For this review, take the finished solid that the model builds, in its own axes (mm). Round coordinates to 2 decimals unless told otherwise and drop trailing zeros. Order: outer loops, then holes, each group sorted by start corner. A loop starts at its lowest first (then second) coordinate and runs counter-clockwise, first axis right, second up. Notation, with made-up numbers: M 61.5,73.25 L 101.5,73.25 A14 cw 101.5,95.25 Z; hole C 31,28 d6. An arc over 180 degrees is marked long. Answer as a JSON object with one key per item and string values.
from build123d import *

# Parameters (mm, degrees)
ESQUISSE1_W        = 100
ESQUISSE1_H        = 82
ESQUISSE1_R        = 1.35
BOSS_EXTRU_1_DEPTH = 2


with BuildPart() as part:
    # Esquisse1 → Boss.-Extru.1 (new body)
    with BuildSketch(Plane.XY.offset(50.5)):
        with Locations((9.361165235, -54.8)):
            Rectangle(ESQUISSE1_W, ESQUISSE1_H)
        with Locations((-36.138834765, -91.3)):
            Circle(ESQUISSE1_R, mode=Mode.SUBTRACT)
        with Locations((-36.138834765, -18.3)):
            Circle(ESQUISSE1_R, mode=Mode.SUBTRACT)
        with Locations((38.861165235, -91.3)):
            Circle(ESQUISSE1_R, mode=Mode.SUBTRACT)
        with Locations((38.861165235, -18.3)):
            Circle(ESQUISSE1_R, mode=Mode.SUBTRACT)
    extrude(amount=BOSS_EXTRU_1_DEPTH)


solid = part.part
1) Add section A-A on y = -91.3. State the section outline as (x, z) points.
Geometry check:
{"outline": "M -40.64,50.5 L -37.49,50.5 L -37.49,52.5 L -40.64,52.5 Z; M -34.79,50.5 L 37.51,50.5 L 37.51,52.5 L -34.79,52.5 Z; M 40.21,50.5 L 59.36,50.5 L 59.36,52.5 L 40.21,52.5 Z"}
2) Insertion check: P1, Ø2.5, axis at x = -36.14, y = -18.3, coming from the +Z side; P2, Ø4.5, axis at x = -36.14, y = -91.3, coming from the +Z side. Each pin has a flat end and moves straight along its axis. Give the tip position at first contact, or say it passes through.
Geometry check:
{"P1": "passes through", "P2": "stops at z = 52.5"}
3) Mouldability with a two-part tool opening along X and no side actions: class faces 1 (the flat face through (9, -54, 50.5)), 2 (the cylindrical face through (-34.851, -17.894, 51.486)), 3 (the flat face through (-40.639, -55, 51)) as +X half, -X half, draft (parallel to the pull), parting line (faces both ways), or undercut.
Geometry check:
{"face 1": "draft", "face 2": "undercut", "face 3": "-X half"}
4) For L1, parallel to X at y = -91.3, z = 50.9, list the stretches that pass through material, from the lowest coordinate up.
Geometry check:
{"L1": "x = -40.64 to -37.49, -34.79 to 37.51, 40.21 to 59.36"}
